Check sheet for the modelled part. Datum: model origin and axes. Units: mm. Face numbers are marked on the shaded views. Give positions to 0.01 mm unless a question says otherwise; leave off trailing zeros. Order: outer loops, then holes, each group sorted by start corner. A loop starts at its lowest first (then second) coordinate and runs counter-clockwise, first axis right, second up.
from build123d import *

# Parameters (mm, degrees)
SKETCH048_W     = 95
SKETCH048_H     = 25
PAD020_DEPTH    = 2.5
SKETCH049_R     = 3.05
PAD021_DEPTH    = 5
SKETCH050_W     = 95
SKETCH050_H     = 25
SKETCH050_W_2   = 89.5
SKETCH050_H_2   = 19.5
POCKET027_DEPTH = 1.25


with BuildPart() as part:
    # Sketch048 → Pad020 (new body)
    with BuildSketch(Plane.XZ):
        with Locations((0, 21.5)):
            Rectangle(SKETCH048_W, SKETCH048_H)
    extrude(amount=PAD020_DEPTH)

    # Sketch049 (on Face5 of Pad020) → Pad021 (join)
    with BuildSketch(Plane(origin=(0, 0, 0), x_dir=(1, 0, 0), z_dir=(0, 1, 0))):
        with Locations((-20, -21.5)):
            Circle(SKETCH049_R)
        with Locations((20, -21.5)):
            Circle(SKETCH049_R)
    extrude(amount=PAD021_DEPTH)

    # Sketch050 (on Face4 of Pad021) → Pocket027 (cut)
    with BuildSketch(Plane(origin=(0, 0, 0), x_dir=(1, 0, 0), z_dir=(0, 1, 0))):
        with Locations((0, -21.5)):
            Rectangle(SKETCH050_W, SKETCH050_H)
        with Locations((0, -21.5)):
            Rectangle(SKETCH050_W_2, SKETCH050_H_2, mode=Mode.SUBTRACT)
    extrude(amount=-POCKET027_DEPTH, mode=Mode.SUBTRACT)


with BuildPart() as part_1:
    # Body010 placement: moved
    add(part.part.moved(Location((0, -70.15, 0))))


solid = part_1.part
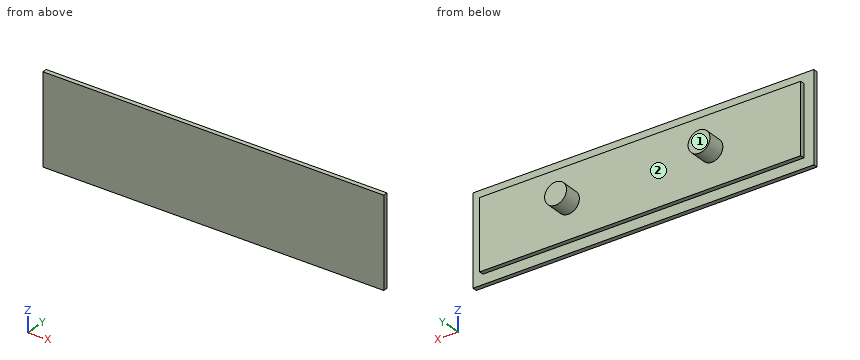
1) Material ranges on L1, parallel to Z at x = -3.5, y = -71.25; L2, parallel to Y at x = -41, z = 22; L3, parallel to Y at x = -42.5, z = 11.25, recorded low to high.
Recorded:
L1: z = 11.75 to 31.25
L2: y = -72.65 to -70.15
L3: y = -72.65 to -71.4
2) Section check D-D, the plane z = 10.5. Record the cut outline in (x, y), then the cut area to 3 significant figures.
Recorded:
outline: (-47.5, -72.65) - (47.5, -72.65) - (47.5, -71.4) - (-47.5, -71.4) - close
area: 119 mm2
3) Section check C-C, the plane y = -67.5. Record the cut outline in (x, z).
Recorded:
outline: circle Ø6.1 at (-20, 21.5); circle Ø6.1 at (20, 21.5)
4) Section check A-A, the plane x = -14. Record the cut outline in (y, z).
Recorded:
outline: (-72.65, 9) - (-71.4, 9) - (-71.4, 11.75) - (-70.15, 11.75) - (-70.15, 31.25) - (-71.4, 31.25) - (-71.4, 34) - (-72.65, 34) - close
5) Depth check by flat-ended pin: pin 1 Ø5 at (x, z) = (36, 13.5) entering from +Y; pin 2 Ø0.6 at (x, y) = (-12.5, -71) entering from -Z; pin 3 Ø0.6 at (y, z) = (-71, 23) entering from +X. Enter the tip coordinate at first touch or a pass-through.
Recorded:
pin 1: stops at y = -70.15
pin 2: stops at z = 11.75
pin 3: stops at x = 44.75
6) Draft check along X on the marked faces 1 and 2. Enter one of: +X half, -X half, draft (parallel to the pull), parting line (faces both ways), or undercut.
Recorded:
face 1: draft
face 2: undercut
7) Section check B-B, the plane z = 21.5. Record the cut outline in (x, y), then the cut area to 3 significant figures.
Recorded:
outline: (-47.5, -72.65) - (47.5, -72.65) - (47.5, -71.4) - (44.75, -71.4) - (44.75, -70.15) - (23.05, -70.15) - (23.05, -65.15) - (16.95, -65.15) - (16.95, -70.15) - (-16.95, -70.15) - (-16.95, -65.15) - (-23.05, -65.15) - (-23.05, -70.15) - (-44.75, -70.15) - (-44.75, -71.4) - (-47.5, -71.4) - close
area: 292 mm2
